Part model, mm, in its own coordinate system. A direction names the side the tool comes from. Give positions to 0.01 mm unless a question says otherwise; leave off trailing zeros. Order: outer loops, then holes, each group sorted by start corner. A loop starts at its lowest first (then second) coordinate and runs counter-clockwise, first axis right, second up. Notation, with made-up numbers: M 27,26.25 L 58,26.25 A9 cw 58,30.25 Z; hole C 3,-34 d11. An arc over 180 degrees is marked long. Answer as a JSON object with one key per item and string values.
Autodesk Inventor part; units mm, degrees
ref_plane "YZ Plane" through (0, 0, 0) normal (1, 0, 0) x (0, 1, 0)
ref_plane "XZ Plane" through (0, 0, 0) normal (0, 1, 0) x (-1, 0, 0)
ref_plane "XY Plane" through (0, 0, 0) normal (0, 0, 1) x (1, 0, 0)
sketch "Sketch1" plane through (0, 0, 0) normal (0, 0, 1) x (1, 0, 0)
  circle A0 centre (50, 87.5) radius 2.01
  circle A1 centre (50, -87.5) radius 2.01
  line L0 (55, -90.5) -> (55, 90.5)
  arc A2 (55, 90.5) -> (53, 92.5) centre (53, 90.5) ccw
  line L1 (53, 92.5) -> (-53, 92.5)
  arc A3 (-53, 92.5) -> (-55, 90.5) centre (-53, 90.5) ccw
  line L2 (-55, 90.5) -> (-55, -90.5)
  arc A4 (-55, -90.5) -> (-53, -92.5) centre (-53, -90.5) ccw
  line L3 (-53, -92.5) -> (53, -92.5)
  arc A5 (53, -92.5) -> (55, -90.5) centre (53, -90.5) ccw
  circle A6 centre (-50, 87.5) radius 2.01
  circle A7 centre (-50, -87.5) radius 2.01
ref_plane "Work Plane1" through (0, 0, 0) normal (0, 0, -1) x (-1, 0, 0)
sketch "Sketch2" plane through (0, 0, 0) normal (0, 0, -1) x (-1, 0, 0)
  arc A0 (42.8653, 89.5) -> (52, 80.3653) centre (55, 92.5) ccw
  line L0 (42.8653, 89.5) -> (-42.8653, 89.5)
  arc A1 (-52, 80.3653) -> (-42.8653, 89.5) centre (-55, 92.5) ccw
  line L1 (-52, 80.3653) -> (-52, -80.3653)
  line L2 (52, -80.3653) -> (52, 80.3653)
  arc A2 (52, -80.3653) -> (42.8653, -89.5) centre (55, -92.5) ccw
  line L3 (-42.8653, -89.5) -> (42.8653, -89.5)
  arc A3 (-42.8653, -89.5) -> (-52, -80.3653) centre (-55, -92.5) ccw
  line L4 (-42.4044, 88.9) -> (42.4044, 88.9)
  arc A4 (42.4044, 88.9) -> (51.4, 79.9044) centre (55, 92.5) ccw
  line L5 (51.4, 79.9044) -> (51.4, -79.9044)
  arc A5 (51.4, -79.9044) -> (42.4044, -88.9) centre (55, -92.5) ccw
  line L6 (42.4044, -88.9) -> (-42.4044, -88.9)
  arc A6 (-42.4044, -88.9) -> (-51.4, -79.9044) centre (-55, -92.5) ccw
  line L7 (-51.4, -79.9044) -> (-51.4, 79.9044)
  arc A7 (-51.4, 79.9044) -> (-42.4044, 88.9) centre (-55, 92.5) ccw
  line L8 (39.6817, 84.9) -> (-39.6817, 84.9)
  arc A8 (-47.4, 77.1817) -> (-39.6817, 84.9) centre (-55, 92.5) ccw
  line L9 (-47.4, 77.1817) -> (-47.4, -77.1817)
  arc A9 (-39.6817, -84.9) -> (-47.4, -77.1817) centre (-55, -92.5) ccw
  line L10 (-39.6817, -84.9) -> (39.6817, -84.9)
  arc A10 (47.4, -77.1817) -> (39.6817, -84.9) centre (55, -92.5) ccw
  line L11 (47.4, -77.1817) -> (47.4, 77.1817)
  arc A11 (39.6817, 84.9) -> (47.4, 77.1817) centre (55, 92.5) ccw
  point P0 (-50, -92.5)
  point P1 (50, -92.5)
  point P2 (50, 92.5)
  point P3 (-50, 92.5)
  dimension "d11" = 0.6
  dimension "d12" = 4
extrude "Extrusion2" add sketch "Sketch2" along normal blind 4 contours L4 A4 L5 A5 L6 A6 L7 A7
extrude "Extrusion3" add sketch "Sketch1" along normal blind 3
properties part number "Tampa caixa principal"
1. Which spindle directions (+Z, -Z, +X, -X, +Y, -Y) get a long thin tool onto all of the face, cutting with end or side? Do faces 4 (the cylindrical face through (-45.671, -83.303, -1.972)), 5 (the cylindrical face through (-45.803, 83.171, -1.972)), 6 (the flat face through (-1, -88.9, -2)), 7 (the flat face through (-51.4, 1, -2)), 8 (the cylindrical face through (42.854, 80.464, -1.972)). Say none if no direction does.
Worked answers:
{"face 4": "-Z, -X, -Y", "face 5": "-Z, -X, +Y", "face 6": "-Z, +X, -X, -Y", "face 7": "-Z, -X, +Y, -Y", "face 8": "-Z"}
2. Two-plate mould, pull along Y, no slides. Class faces 1 (the flat face through (-47.4, -1, -2)), 2 (the flat face through (-1, 1, 3)), 3 (the cylindrical face through (45.671, 83.303, -1.972)): +Y half, -Y half, draft (parallel to the pull), parting line (faces both ways), or undercut.
Worked answers:
{"face 1": "undercut", "face 2": "draft", "face 3": "+Y half"}
3. Pin check, flat tips, straight feed: P1, Ø2, axis at y = -23.5, z = -2.5, coming from the +X side; P2, Ø4.5, axis at x = 50, y = -87.5, coming from the +Z side; P3, Ø2, axis at y = -35.5, z = -2, coming from the -X side; P4, Ø1, axis at x = 35, z = -1, coming from the -Y side. Stop position of each tip, or through.
Worked answers:
{"P1": "stops at x = 51.4", "P2": "stops at z = 3", "P3": "stops at x = -51.4", "P4": "stops at y = -88.9"}
4. Cut at B-B on x = 24. Give the cut face in (y, z).
Worked answers:
{"outline": "M -92.5,0 L -88.9,0 L -88.9,-4 L -84.9,-4 L -84.9,0 L 84.9,0 L 84.9,-4 L 88.9,-4 L 88.9,0 L 92.5,0 L 92.5,3 L -92.5,3 Z"}
5. Cut at A-A on z = -1.25. Give the cut face in (x, y).
Worked answers:
{"outline": "M -51.4,-79.9 A13.1 cw -42.4,-88.9 L 42.4,-88.9 A13.1 cw 51.4,-79.9 L 51.4,79.9 A13.1 cw 42.4,88.9 L -42.4,88.9 A13.1 cw -51.4,79.9 Z; hole M -47.4,-77.18 A17.1 cw -39.68,-84.9 L 39.68,-84.9 A17.1 cw 47.4,-77.18 L 47.4,77.18 A17.1 cw 39.68,84.9 L -39.68,84.9 A17.1 cw -47.4,77.18 Z"}
6. Cut at C-C on y = -74. Give the cut face in (x, z), plus the area to 3 significant figures.
Worked answers:
{"outline": "M -55,0 L -51.4,0 L -51.4,-4 L -47.4,-4 L -47.4,0 L 47.4,0 L 47.4,-4 L 51.4,-4 L 51.4,0 L 55,0 L 55,3 L -55,3 Z", "area": "362 mm^2"}
7. Probe line 1 along Y through (x, z) = (-50, 1.5); line 2 along X through (y, z) = (-75.5, -1.75); line 3 along Y through (x, z) = (35, -1.25). List the from-to ranges inside material, lowest first.
Worked answers:
{"line 1": "y = -92.5 to -89.51, -85.49 to 85.49, 89.51 to 92.5", "line 2": "x = -51.4 to -47.4, 47.4 to 51.4", "line 3": "y = -88.9 to -84.9, 84.9 to 88.9"}
